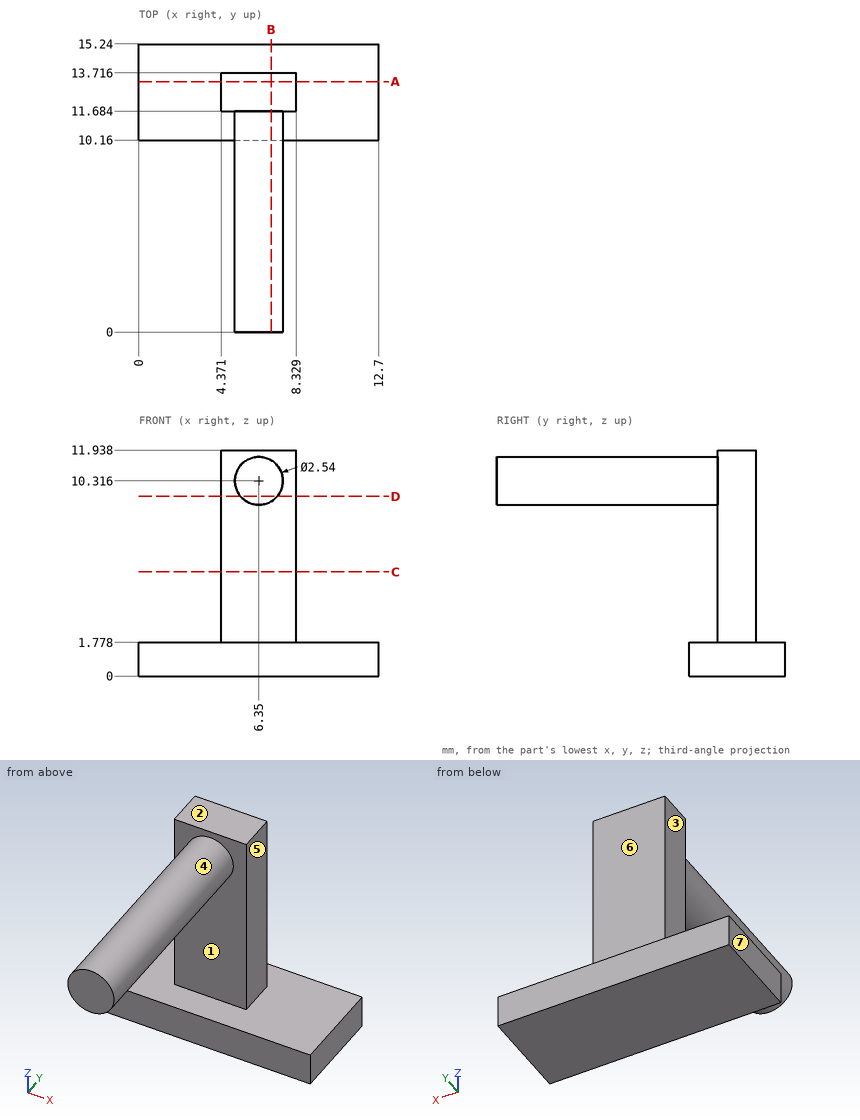
Verification items for this drawing (mm, ordinates from the low corner). A direction names the side the tool comes from. Round coordinates to 2 decimals unless told otherwise and drop trailing zeros. Loops run counter-clockwise (first coordinate to the right, second up) from the corner with the lowest first, then second, coordinate; pieces in that order, holes last. Notation, with made-up numbers: M 55.25,-14 L 77.25,-14 A7 ccw 77.25,-6 Z; hole C 36.25,77.25 d4. An arc over 180 degrees is marked long. Answer as a JSON object with one key per item and string values.
1. Mould release check, pull along Z, two halves, no side actions. Record for the marked faces 1, 2 and 3: pulls with the +Z half, pulls with the -Z half, needs draft (parallel to the pull), parting line crosses it, or undercut.
Reply:
{"face 1": "undercut", "face 2": "pulls with the +Z half", "face 3": "needs draft"}
2. Section check D-D (z = 9.5). Record the boundary of the cut face in (x, y).
Reply:
{"outline": "M 4.37,11.68 L 5.38,11.68 L 5.38,0 L 7.32,0 L 7.32,11.68 L 8.33,11.68 L 8.33,13.72 L 4.37,13.72 Z"}
3. Gauge pin test, flat ends, axial feed: P1, Ø1.5, axis at x = 7, z = 9.5, coming from the -Y side; P2, Ø6, axis at x = 7.5, z = 6, coming from the -Y side; P3, Ø4, axis at x = 10.5, z = 5.5, coming from the -Y side; P4, Ø1.6, axis at y = 12.5, z = 4.5, coming from the +X side. Record the tip position at first contact, or that the pin passes through.
Reply:
{"P1": "stops at y = 0", "P2": "stops at y = 11.68", "P3": "passes through", "P4": "stops at x = 8.33"}
4. Section check A-A (y = 13.25). Record the boundary of the cut face in (x, z).
Reply:
{"outline": "M 0,0 L 12.7,0 L 12.7,1.78 L 8.33,1.78 L 8.33,11.94 L 4.37,11.94 L 4.37,1.78 L 0,1.78 Z"}
5. Access from +Z, -Z, +X, -X, +Y, -Y to the whole of each face (thin tool, end or side, straight path). Record for the marked faces 4, 5, 6 and 7.
Reply:
{"face 4": "-Y", "face 5": "+Z, +X, +Y, -Y", "face 6": "+Z, +X, -X, +Y", "face 7": "+Z, -Z, -X, +Y, -Y"}
6. Scan lines: line 1 (X direction, y = 12.5, z = 7); line 2 (Y direction, x = 5, z = 11.25); line 3 (Z direction, x = 1.75, y = 14.5). Record each from-to range of solid material in increasing order.
Reply:
{"line 1": "x = 4.37 to 8.33", "line 2": "y = 11.68 to 13.72", "line 3": "z = 0 to 1.78"}
7. Section check B-B (x = 7). Record the boundary of the cut face in (y, z) (1 decimal).
Reply:
{"outline": "M 0,9.2 L 11.7,9.2 L 11.7,1.8 L 10.2,1.8 L 10.2,0 L 15.2,0 L 15.2,1.8 L 13.7,1.8 L 13.7,11.9 L 11.7,11.9 L 11.7,11.4 L 0,11.4 Z"}
8. Section check C-C (z = 5.5). Record the boundary of the cut face in (x, y).
Reply:
{"outline": "M 4.37,11.68 L 8.33,11.68 L 8.33,13.72 L 4.37,13.72 Z"}
